Autodesk Inventor part; units mm, degrees
ref_plane "YZ Plane" through (0, 0, 0) normal (1, 0, 0) x (0, 1, 0)
ref_plane "XZ Plane" through (0, 0, 0) normal (0, 1, 0) x (-1, 0, 0)
ref_plane "XY Plane" through (0, 0, 0) normal (0, 0, 1) x (1, 0, 0)
sketch "Sketch1" plane through (0, 0, 0) normal (0, 0, 1) x (1, 0, 0)
  line L0 (0, 0) -> (0, 40) construction
  line L1 (0, 40) -> (-420, 40) construction
  line L2 (-420, 0) -> (-420, 40) construction
  line L3 (0, 0) -> (-420, 0) construction
  line L4 (40, 120) -> (0, 120) construction
  line L5 (0, 120) -> (0, -730) construction
  line L6 (40, -730) -> (0, -730) construction
  line L7 (40, 120) -> (40, -730) construction
  line L8 (0, 0) -> (40, 0) construction
  line L9 (40, 0) -> (40, 40) construction
  line L10 (40, 40) -> (0, 40) construction
  line L11 (0, 40) -> (0, 0) construction
  line L12 (0, 0) -> (-60, 0) construction
  line L13 (-60, 0) -> (-60, 40) construction
  line L14 (-60, 40) -> (0, 40) construction
  line L15 (0, 40) -> (0, 0) construction
  line L16 (-23.6304, 41.0957) -> (-1.8765, 58.4988) construction
  line L17 (0, 40) -> (40, 40) construction
  line L18 (40, 40) -> (40, 60) construction
  line L19 (40, 60) -> (0, 60) construction
  line L20 (0, 60) -> (0, 40) construction
  line L21 (-1.8765, 58.4988) -> (0, 60) construction
  line L22 (-23.6304, 41.0957) -> (-25, 40) construction
  line L23 (40, 0) -> (0, 0) construction
  line L24 (0, 0) -> (0, -20) construction
  line L25 (0, -20) -> (40, -20) construction
  line L26 (40, -20) -> (40, 0) construction
  line L27 (-25, 40) -> (-25, 0) construction
  line L28 (-25, 0) -> (0, -20) construction
  line L29 (20, -20) -> (20, 60) construction
  line L30 (0, 20) -> (-60, 20) construction
  line L31 (30, 10) -> (10, 10) construction
  line L32 (10, 10) -> (10, -10) construction
  line L33 (10, -10) -> (30, -10) construction
  line L34 (30, -10) -> (30, 10) construction
  line L35 (30, 10) -> (10, -10) construction
  line L36 (10, 10) -> (30, -10) construction
  line L37 (30, 30) -> (10, 30) construction
  line L38 (10, 30) -> (10, 50) construction
  line L39 (10, 50) -> (30, 50) construction
  line L40 (30, 50) -> (30, 30) construction
  line L41 (30, 30) -> (10, 50) construction
  line L42 (10, 30) -> (30, 50) construction
  line L43 (0, -20) -> (-25, 0)
  line L44 (-25, 0) -> (-60, 0)
  line L45 (-60, 0) -> (-60, 40)
  line L46 (-60, 40) -> (-25, 40)
  line L47 (-25, 40) -> (0, 60)
  line L48 (0, 60) -> (40, 60)
  line L49 (40, 60) -> (40, -20)
  line L50 (40, -20) -> (0, -20)
  line L51 (-30, 20) -> (-45, 20)
  line L52 (-30, 20) -> (-15, 20)
  point P0 (20, 0)
  point P1 (20, 0)
  point P2 (20, 40)
  point P3 (20, 30)
  point P4 (20, 10)
  point P5 (20, -10)
  dimension "d0" = 60
  dimension "d1" = 40
  dimension "d2" = 20
  dimension "d3" = 20
  dimension "d6" = 20
  dimension "d7" = 20
  dimension "d8" = 20
  dimension "d9" = 20
  dimension "d20" = 15
  dimension "d21" = 15
extrude "Extrusion1" add sketch "Sketch1" along normal blind 3
hole "Hole1" at (20, -10, 0) at (20, 10, 0) at (20, 30, 0) direction (0, 0, 1) diameter 5 depth 8 tip angle 118
fillet "Fillet1" radius 5 2 edges at (-25, 40, 1.5) (-25, 0, 1.5)
hole "Hole2" at (-45, 20, 0) at (-15, 20, 0) direction (0, 0, 1) diameter 5 depth 8 tip angle 118
sketch "Sketch2" plane through (0, 0, 3) normal (0, 0, 1) x (1, 0, 0)
  circle A0 centre (-45, 20) radius 2.5
  circle A1 centre (-15, 20) radius 2.5
  line L0 (40, -20) -> (40, 60)
  line L1 (40, 60) -> (0, 60)
  line L2 (0, 60) -> (-23.6304, 41.0957)
  arc A2 (-26.7539, 40) -> (-23.6304, 41.0957) centre (-26.7539, 45) ccw
  line L3 (-26.7539, 40) -> (-60, 40)
  line L4 (-60, 40) -> (-60, 0)
  line L5 (-60, 0) -> (-26.7539, 0)
  arc A3 (-23.6304, -1.0957) -> (-26.7539, 0) centre (-26.7539, -5) ccw
  line L6 (-23.6304, -1.0957) -> (0, -20)
  line L7 (0, -20) -> (40, -20)
  line L8 (-26.7539, 40) -> (-60, 40)
  line L9 (-26.7539, 40) -> (40, 40)
  point P0 (0, 0)
extrude "Extrusion2" cut sketch "Sketch2" against normal blind 3 contours L9 A2 L2 L1 L0
properties part number "bigusset"
Design review of the part built by this model. Coordinates are the model's own, in mm. A direction names the side the tool comes from. Give positions to 0.01 mm unless a question says otherwise; leave off trailing zeros. Loops run counter-clockwise (first coordinate to the right, second up) from the corner with the lowest first, then second, coordinate; pieces in that order, holes last. Notation, with made-up numbers: M 73.25,81 L 120.25,81 A23 cw 120.25,102 Z; hole C -2,-6.75 d9. An arc over 180 degrees is marked long. Answer as a JSON object with one key per item and string values.
Item 1: Wall thickness on line 1 along Y through (x, z) = (20, 0.65); line 2 along X through (y, z) = (20, 2.35); line 3 along X through (y, z) = (10, 1.25): over which ranges is each line inside the solid? List them lowest first.
Output values:
{"line 1": "y = -20 to -12.5, -7.5 to 7.5, 12.5 to 27.5, 32.5 to 40", "line 2": "x = -60 to -47.5, -42.5 to -17.5, -12.5 to 40", "line 3": "x = -60 to 17.5, 22.5 to 40"}
Item 2: We need section A-A (x = -15). State the section outline as (y, z) points, and give its area (3 significant figures).
Output values:
{"outline": "M -8,0 L 17.5,0 L 17.5,3 L -8,3 Z; M 22.5,0 L 40,0 L 40,3 L 22.5,3 Z", "area": "129 mm2"}
Item 3: Mouldability with a two-part tool opening along Y and no side actions: class faces 3 (the face through (-11, 40, 1)), 4 (the face through (17.52, 9.67, 1.52)), 5 (the face through (-25.08, -0.29, 1.52)) as pulls with the +Y half, pulls with the -Y half, needs draft (parallel to the pull), parting line crosses it, or undercut.
Output values:
{"face 3": "pulls with the +Y half", "face 4": "undercut", "face 5": "pulls with the -Y half"}
Item 4: We need section B-B (y = 20). State the section outline as (x, z) points.
Output values:
{"outline": "M -60,0 L -47.5,0 L -47.5,3 L -60,3 Z; M -42.5,0 L -17.5,0 L -17.5,3 L -42.5,3 Z; M -12.5,0 L 40,0 L 40,3 L -12.5,3 Z"}
Item 5: We need section C-C (z = 2.4). State the section outline as (x, y) points, and give its area (3 significant figures).
Output values:
{"outline": "M -60,0 L -26.75,0 A5 cw -23.63,-1.1 L 0,-20 L 40,-20 L 40,40 L -60,40 Z; hole C -45,20 d5; hole C -15,20 d5; hole C 20,-10 d5; hole C 20,10 d5; hole C 20,30 d5", "area": "4,950 mm2"}
Item 6: We need section D-D (y = -10). State the section outline as (x, z) points, and give its area (4 significant figures).
Output values:
{"outline": "M -12.5,0 L 17.5,0 L 17.5,3 L -12.5,3 Z; M 22.5,0 L 40,0 L 40,3 L 22.5,3 Z", "area": "142.5 mm2"}
Item 7: Machinability: for faces 1 (the face through (-43, 0, 1)), 2 (the face through (17.52, -10.33, 1.52)), which of the approach directions +Z, -Z, +X, -X, +Y, -Y give a long, thin tool a straight path to every point of the face, cutting with its end or side? Answer none if there is none.
Output values:
{"face 1": "+Z, -Z, -X, -Y", "face 2": "+Z, -Z"}
Item 8: For P1, Ø1, axis at x = -20, y = 29.5, coming from the -Z side; P2, Ø4, axis at x = 20, y = -10, coming from the -Z side, all flat-tipped, find the tip position at first contact; note any pin that passes through.
Output values:
{"P1": "stops at z = 0", "P2": "passes through"}
